Input: part model. Units: mm. Frame: model coordinates. A direction names the side the tool comes from. Give positions to 0.01 mm unless a question says otherwise; leave off trailing zeros. Loops run counter-clockwise (first coordinate to the right, second up) from the corner with the lowest first, then second, coordinate; pieces in that order, holes last. Notation, with made-up numbers: M 10,-33.75 L 50,-33.75 A20 cw 50,-8.75 Z; hole C -39.5,72 d4. An arc over 180 degrees is marked long. Answer as a JSON object with one key per item and string values. Group by question number.
```python
from build123d import *

# Parameters (mm, degrees)
F1_DEPTH     = 20
F2_W         = 14
F2_H         = 63
F3_DEPTH     = 25
F4_W         = 28
F4_H         = 22
F5_DEPTH     = 25
F7_DEPTH     = 16
F10_DEPTH    = 17
F9_R         = 21
F11_DEPTH    = 10
F13_SIZE     = 2
F14_T1_DEPTH = 30.2867319519
F14_T3_DEPTH = 26.2867319519
F14_T5_DEPTH = 25.9668324626
F15_SIZE     = 2
F18_W        = 68.8039958477
F18_H        = 47.8929802775
F19_DEPTH    = 10


# Not quite as in the source:
# - a fillet or chamfer that OpenCascade refuses, or shapes differently, is made with other operations: its cross-section is extruded or revolved along the edge and cut away or added


with BuildPart() as f1:
    # F0 (on Front) → F1 (new body)
    with BuildSketch(Plane.XZ):
        Polygon((-30.5923320651, 260.9896056354), (-146.5923320651, 260.9896056354), (-146.5923320651, -39.0103943646), (-112.5923320651, -39.0103943646), (-30.5923320651, -39.0103943646), align=None)
        Polygon((-30.5923320651, -49.0103943646), (-30.5923320651, -39.0103943646), (-112.5923320651, -39.0103943646), (-112.5923320651, -49.0103943646), (-92.5923320651, -49.0103943646), (-50.5923320651, -49.0103943646), align=None)
    extrude(amount=-F1_DEPTH)

    # F2 (on face) → F3 (cut)
    with BuildSketch(Plane.XZ):
        Polygon((-158.5923320651, 124.9896056354), (-158.5923320651, -39.0103943646), (-98.5923320651, -39.0103943646), (-98.5923320651, 106.9896056354), (-98.5923320651, 124.9896056354), align=None)
        Polygon((-98.5923320651, 124.9896056354), (-98.5923320651, 106.9896056354), (-62.5923320651, 106.9896056354), (-62.5923320651, 124.9896056354), (-76.5923320651, 124.9896056354), align=None)
        with Locations((-69.5923320651, 156.4896056354)):
            Rectangle(F2_W, F2_H)
        with BuildLine():
            ThreePointArc((-62.5923320651, 187.9896056354), (-69.5923320651, 194.9896056354), (-76.5923320651, 187.9896056354))
            Line((-76.5923320651, 187.9896056354), (-62.5923320651, 187.9896056354))
        make_face()
        Polygon((-146.5923320651, 260.9896056354), (-146.5923320651, 178.9896056354), (-96.5923320651, 260.9896056354), align=None)
    extrude(amount=-F3_DEPTH, mode=Mode.SUBTRACT)

    # F4 (on face) → F5 (cut)
    with BuildSketch(Plane.XZ):
        with Locations((-74.5923320651, 231.9896056354)):
            Rectangle(F4_W, F4_H)
        with BuildLine():
            ThreePointArc((-60.5923320651, 220.9896056354), (-49.5923320651, 231.9896056354), (-60.5923320651, 242.9896056354))
            Line((-60.5923320651, 242.9896056354), (-60.5923320651, 220.9896056354))
        make_face()
        with BuildLine():
            Line((-88.5923320651, 220.9896056354), (-88.5923320651, 242.9896056354))
            ThreePointArc((-88.5923320651, 242.9896056354), (-99.5923320651, 231.9896056354), (-88.5923320651, 220.9896056354))
        make_face()
    extrude(amount=-F5_DEPTH, mode=Mode.SUBTRACT)

    # F6 (on face) → F7 (join)
    with BuildSketch(Plane.XZ):
        Polygon((-30.5923320651, -39.0103943646), (-98.5923320651, -39.0103943646), (-112.5923320651, -39.0103943646), (-112.5923320651, -49.0103943646), (-30.5923320651, -49.0103943646), align=None)
    extrude(amount=F7_DEPTH)

    # F8 (on face) → F10 (join)
    with BuildSketch(Plane(origin=(0, 20, 0), x_dir=(-1, 0, 0), z_dir=(0, 1, 0))):
        Polygon((112.5923320651, -39.0103943646), (98.5923320651, -39.0103943646), (30.5923320651, -39.0103943646), (30.5923320651, -49.0103943646), (112.5923320651, -49.0103943646), align=None)
    extrude(amount=F10_DEPTH)

    # F9 (on face) → F11 (join)
    with BuildSketch(Plane(origin=(0, 0, -49.0103943646), x_dir=(1, 0, 0), z_dir=(0, 0, -1))):
        with Locations((-71.5923320651, -10)):
            Circle(F9_R)
    extrude(amount=F11_DEPTH)

    # F13
    f13_edges = [f1.edges().sort_by_distance(p)[0] for p in [
        (-98.592332, 0, 33.989606),
        (-98.592332, 20, 33.989606),
    ]]
    chamfer(f13_edges, length=F13_SIZE)

    # F14: chamfer of 2 on 4 edges, made by hand

    # F14_s2 → F14_t1 (cut)
    with BuildSketch(Plane.XZ.offset(-25.1433659759)):
        Polygon((-146.5923320651, 126.9896056354), (-144.5923320651, 124.9896056354), (-146.5923320651, 124.9896056354), align=None)
        Polygon((-76.5923320651, 126.9896056354), (-78.5923320651, 124.9896056354), (-76.5923320651, 124.9896056354), align=None)
    extrude(amount=F14_T1_DEPTH, mode=Mode.SUBTRACT)

    # F14_s4 → F14_t3 (cut)
    with BuildSketch(Plane.XZ.offset(-23.1433659759)):
        Polygon((-96.5923320651, 106.9896056354), (-98.5923320651, 104.9896056354), (-98.5923320651, 106.9896056354), align=None)
    extrude(amount=F14_T3_DEPTH, mode=Mode.SUBTRACT)

    # F14_s6 → F14_t5 (cut)
    with BuildSketch(Plane.XZ.offset(-22.9834162313)):
        Polygon((-95.4693648059, 260.9896056354), (-97.1769571575, 260.0308204839), (-96.5923320651, 260.9896056354), align=None)
    extrude(amount=F14_T5_DEPTH, mode=Mode.SUBTRACT)

    # F15
    f15_edges = [f1.edges().sort_by_distance(p)[0] for p in [
        (-111.592332, 0, 124.989606),
        (-111.592332, 20, 124.989606),
        (-79.592332, 0, 106.989606),
        (-79.592332, 20, 106.989606),
        (-63.030848, 0, 260.989606),
        (-63.030848, 20, 260.989606),
    ]]
    chamfer(f15_edges, length=F15_SIZE)

    # F18 (on face) → F19 (join)
    with BuildSketch(Plane(origin=(0, 107.4948028177, 107.4948028177), x_dir=(1, 0, 0), z_dir=(0, -0.7071067812, -0.7071067812))):
        with Locations((-111.8147820234, 100.1271270216)):
            Rectangle(F18_W, F18_H)
    extrude(amount=F19_DEPTH)


solid = f1.part
```
1. Reachability of faces 1 (the cylindrical face through (-92.572, 9.077, -53.94)), 2 (the flat face through (-98.592, 10, 32)), 3 (the flat face through (-75, 10, 242.99)) from +Z, -Z, +X, -X, +Y, -Y: full face, straight path, thin tool, end or side. Return the list, or none.
2. First-contact query: P1, Ø1, axis at x = -58.5, z = 195.5, coming from the -Y side; P2, Ø8, axis at y = 12, z = 35.5, coming from the -X side; P3, Ø6, axis at x = -59.5, z = 24.5, coming from the +Y side; P4, Ø20.5, axis at y = 26.5, z = 172.5, coming from the -X side. Flat tips, straight axial feed; report the tip coordinate or a pass-through.
3. Material intervals for L1, parallel to Z at x = -95, y = 7; L2, parallel to X at y = 4.5, z = 91; L3, parallel to Z at x = -95, y = -0.5, sorted ascending.
4. Mould query, pull axis X, two halves, no side actions, for faces 4 (the flat face through (-75, 10, 220.99)), 5 (the flat face through (-112.296, 50.141, 157.877)), 6 (the flat face through (-62.592, 10, 146)), 7 (the flat face through (-146.217, 33, 175)). Classes: pulls with the +X half, pulls with the -X half, needs draft (parallel to the pull), parting line crosses it, or undercut.
5. Section C-C (x = -123.5). Output: boundary loops of the cut face in (y, z).
6. Section B-B (z = 72). Output: boundary loops of the cut face in (x, y), then the cut area to 3 significant figures.
7. Section A-A (y = -6). Output: boundary loops of the cut face in (x, z), then the cut area to 3 significant figures.
Geometry results:
{
 "1": {"face 1": "-Z", "face 2": "-X, +Y, -Y", "face 3": "+Y, -Y"},
 "2": {"P1": "y = 0", "P2": "x = -98.59", "P3": "y = 20", "P4": "x = -146.59"},
 "3": {"L1": "-49.01 to 106.99, 124.99 to 223.05, 240.93 to 260.99", "L2": "-98.59 to -30.59", "L3": "-49.01 to -39.01"},
 "4": {"face 4": "undercut", "face 5": "needs draft", "face 6": "undercut", "face 7": "pulls with the -X half"},
 "5": {"outline": "M 0,126.99 L 2,124.99 L 18,124.99 L 20,126.99 L 20,180.85 L 46.56,154.29 L 53.63,161.36 L 20,194.99 L 20,216.86 L 0,216.86 Z"},
 "6": {"outline": "M -98.59,2 L -96.59,0 L -30.59,0 L -30.59,20 L -96.59,20 L -98.59,18 Z", "area": "1,360 mm2"},
 "7": {"outline": "M -112.59,-49.01 L -85.19,-49.01 L -85.19,-59.01 L -57.99,-59.01 L -57.99,-49.01 L -30.59,-49.01 L -30.59,-39.01 L -112.59,-39.01 Z", "area": "1,090 mm2"}
}
